Input: part model. Units: mm. Frame: model coordinates. A direction names the side the tool comes from. Coordinates: 2 decimals unless noted, no trailing zeros. Loops run counter-clockwise (first coordinate to the right, second up) from the corner with the lowest first, then second, coordinate; pieces in that order, holes last.
Item 1: Section C-C on y = 1.75. Return loops of the section in (x, z).
Item 2: Ray query, line 1 along Z through (x, y) = (3.5, 2.4); line 2 along Z through (x, y) = (3.5, 0.8); line 3 along X through (y, z) = (1.45, -18.75). Return the intervals inside material, ascending.
Item 3: Reachability of faces 5 (the cylindrical face through (2.42, 1.52, 19.93)), 6 (the flat face through (4, 3, -17)) from +Z, -Z, +X, -X, +Y, -Y: full face, straight path, thin tool, end or side. Return the list, or none.
Item 4: Pull-direction query (Z, two-part tool) for faces 1 (the cylindrical face through (3.451, 12.247, 0.269)), 2 (the cylindrical face through (3.451, 15.247, 0.293)), 3 (the flat face through (4, 2, -22.25)), 4 (the flat face through (4, 3, 17)); classes: released by +Z, released by -Z, zero draft, split by the parting line, or undercut.
Item 5: Section B-B on x = 3.5. Return loops of the section in (y, z).
Item 6: Section A-A on z = 18.75. Return loops of the section in (x, y).
Item 7: Contact query for flat-ended pins moving along their axis: P1, Ø3.5, axis at x = 3, z = -17.5, coming from the +Y side; P2, Ø2, axis at x = 5.5, z = 3.5, coming from the -Y side; P3, Ø1.5, axis at x = 6.5, z = 4.5, coming from the -Y side. Output: stop coordinate, or through.
Item 8: Section D-D on y = 6.75. Return loops of the section in (x, z).
Autodesk Inventor part; units mm, degrees
ref_plane "YZ Plane" through (0, 0, 0) normal (1, 0, 0) x (0, 1, 0)
ref_plane "XZ Plane" through (0, 0, 0) normal (0, 1, 0) x (-1, 0, 0)
ref_plane "XY Plane" through (0, 0, 0) normal (0, 0, 1) x (1, 0, 0)
sketch "Skizze1" plane through (0, 0, 0) normal (1, 0, 0) x (0, 1, 0)
  arc A0 (0, -12.25) -> (0, 12.25) centre (0, 0) ccw
  line L0 (0, 0) -> (0, 12.25) construction
  line L1 (0, 0) -> (0, -12.25) construction
  arc A1 (0, -15.25) -> (0, 15.25) centre (0, 0) ccw
  line L2 (0, 15.25) -> (0, 12.25)
  line L3 (0, -12.25) -> (0, -15.25)
  dimension "d0" = 12.25
  dimension "d1" = 180
  dimension "d3" = 15.25
extrude "Extrusion1" add sketch "Skizze1" along normal blind 7
sketch "Skizze3" plane through (7, 0, 0) normal (1, 0, 0) x (0, 0, -1)
  arc A0 (15.25, 0) -> (-15.25, 0) centre (0, 0) ccw
  line L0 (-15.25, 0) -> (-22.25, 0)
  line L1 (-22.25, 0) -> (-22.25, 3)
  line L2 (-22.25, 3) -> (-14.952, 3)
  dimension "d6" = 7
  dimension "d7" = 3
extrude "Extrusion3" add sketch "Skizze3" against normal blind 7
sketch "Skizze5" plane through (0, 0, 12.25) normal (0, -1, 0) x (1, 0, 0)
  line L0 (7, 10) -> (7, 0)
  line L1 (7, 10) -> (0, 10)
  point P0 (0, -12.25)
  point P1 (3.5, 6.5)
  dimension "d19" = 3.5
  dimension "d20" = 3.5
hole "Bohrung1" at (3.5, 0, 18.75) direction (0, 1, 0) diameter 3.2 end through all
mirror "Spiegeln1" about plane through (0, 0, 0) normal (0, 0, 1) of "Extrusion3", "Bohrung1"
properties part number "klemme"
Results found:
1. outline: (0, -22.25) - (7, -22.25) - (7, -12.12) - (0, -12.12) - close; (0, 12.12) - (7, 12.12) - (7, 22.25) - (0, 22.25) - close; hole circle Ø3.2 at (3.5, -18.75); hole circle Ø3.2 at (3.5, 18.75)
2. line 1: z = -22.25 to -20.35, -17.15 to -12.01, 12.01 to 17.15, 20.35 to 22.25
2. line 2: z = -22.25 to -20.35, -17.15 to -12.22, 12.22 to 17.15, 20.35 to 22.25
2. line 3: x = 0 to 1.9, 5.1 to 7
3. face 5: +Y, -Y
3. face 6: -Z, +X, -X, +Y
4. face 1: undercut
4. face 2: split by the parting line
4. face 3: released by -Z
4. face 4: zero draft
5. outline: (0, -22.25) - (3, -22.25) - (3, -20.35) - (0, -20.35) - close; (0, -17.15) - (3, -17.15) - (3, -14.95) arc R15.25 ccw to (3, 14.95) - (3, 17.15) - (0, 17.15) - (0, 12.25) arc R12.25 cw to (0, -12.25) - close; (0, 20.35) - (3, 20.35) - (3, 22.25) - (0, 22.25) - close
6. outline: (0, 0) - (1.9, 0) - (1.9, 3) - (0, 3) - close; (5.1, 0) - (7, 0) - (7, 3) - (5.1, 3) - close
7. P1: stops at y = 3
7. P2: stops at y = 11.39
7. P3: stops at y = 11.07
8. outline: (0, -13.67) - (7, -13.67) - (7, -10.22) - (0, -10.22) - close; (0, 10.22) - (7, 10.22) - (7, 13.67) - (0, 13.67) - close
